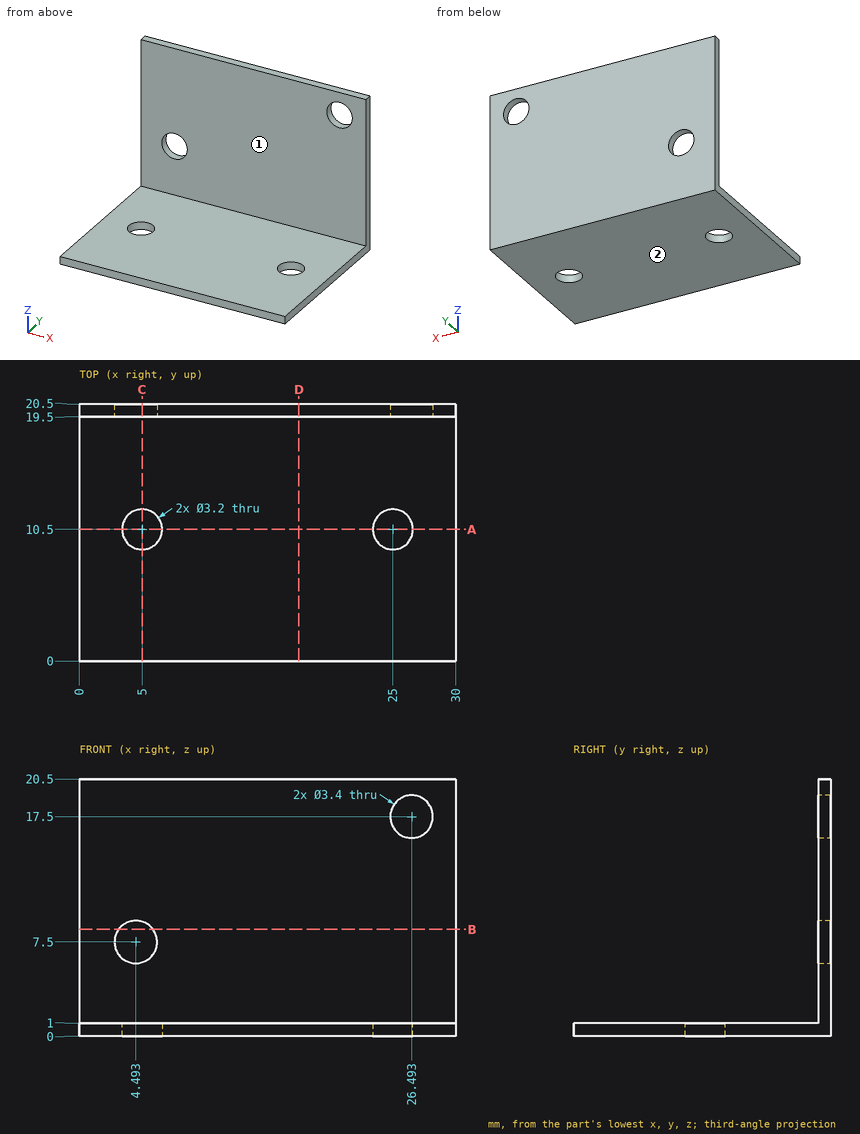
Verification items for this drawing (mm, ordinates from the low corner). A direction names the side the tool comes from. Coordinates: 2 decimals unless noted, no trailing zeros. Order: outer loops, then holes, each group sorted by start corner. A loop starts at its lowest first (then second) coordinate and runs counter-clockwise, first axis right, second up. Notation, with made-up numbers: (-26, -35.5) -> (-21, -35.5) arc R21 ccw to (-21, -9.5) -> close; hole circle Ø6 at (-22, -12.75). An arc over 180 degrees is marked (long way). Put each result on its own line as item: value. Start each with the question number.
1. Cross-section at D-D, the plane x = 17.5. Record the boundary of the cut face in (y, z).
2. Access from +Z, -Z, +X, -X, +Y, -Y to the whole of each face (thin tool, end or side, straight path). Record for the marked faces 1 and 2.
3. Cross-section at C-C, the plane x = 5. Record the boundary of the cut face in (y, z).
4. Cross-section at A-A, the plane y = 10.5. Record the boundary of the cut face in (x, z).
5. Material ranges on L1, parallel to X at y = 19.7, z = 17.5; L2, parallel to Y at x = 5, z = 0.4; L3, parallel to Z at x = 17.25, y = 17, recorded low to high. Write a range as [from, to].
6. Go/stop test with flat-tipped pins: pin 1 Ø6 at (x, z) = (16.5, 9) entering from -Y; pin 2 Ø2.5 at (x, z) = (4.49, 7.5) entering from +Y. Record where each tip stops, or that it passes through.
7. Cross-section at B-B, the plane z = 8.5. Record the boundary of the cut face in (x, y).
Computed:
1. outline: (0, 0) -> (20.5, 0) -> (20.5, 20.5) -> (19.5, 20.5) -> (19.5, 1) -> (0, 1) -> close
2. face 1: +Z, +X, -X, -Y
2. face 2: -Z, +X, -X, +Y, -Y
3. outline: (0, 0) -> (8.9, 0) -> (8.9, 1) -> (0, 1) -> close; (12.1, 0) -> (20.5, 0) -> (20.5, 5.88) -> (19.5, 5.88) -> (19.5, 1) -> (12.1, 1) -> close; (19.5, 9.12) -> (20.5, 9.12) -> (20.5, 20.5) -> (19.5, 20.5) -> close
4. outline: (0, 0) -> (3.4, 0) -> (3.4, 1) -> (0, 1) -> close; (6.6, 0) -> (23.4, 0) -> (23.4, 1) -> (6.6, 1) -> close; (26.6, 0) -> (30, 0) -> (30, 1) -> (26.6, 1) -> close
5. L1: [0, 24.79], [28.19, 30]
5. L2: [0, 8.9], [12.1, 20.5]
5. L3: [0, 1]
6. pin 1: y = 19.5
6. pin 2: through
7. outline: (0, 19.5) -> (3.12, 19.5) -> (3.12, 20.5) -> (0, 20.5) -> close; (5.87, 19.5) -> (30, 19.5) -> (30, 20.5) -> (5.87, 20.5) -> close
